Design review of the part built by this model. Coordinates are the model's own, in mm. Give positions to 0.01 mm unless a question says otherwise; leave off trailing zeros. Write each loop counter-clockwise with the first axis right and the second up, starting at its lowest first coordinate (ties: lowest second). Pieces come first, ordered by that corner, then holes. Notation, with made-up numbers: (-40, 30) -> (-15, 30) arc R14 ccw to (-15, 37) -> close; hole circle Ø11 at (15, 74). An arc over 180 degrees is marked (long way). Answer as a JSON object with one key per item and string values.
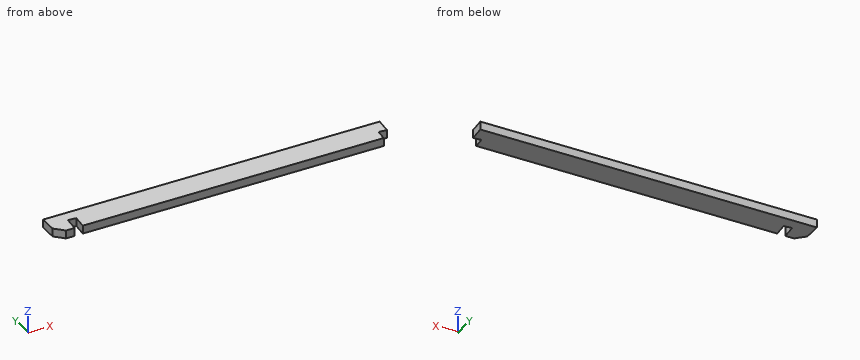
```python
from build123d import *

# Parameters (mm, degrees)
SKETCH1_W           = 47
SKETCH1_H           = 150
BOSS_EXTRUDE1_DEPTH = 1955
CUT_EXTRUDE1_DEPTH  = 1958.002554929
CHAMFER1_SIZE       = 50
CUT_EXTRUDE2_DEPTH  = 1958.002554929
CUT_EXTRUDE3_DEPTH  = 1958.002554929


with BuildPart() as part:
    # Sketch1 → Boss-Extrude1 (new body)
    with BuildSketch(Plane(origin=(0, 0, 0), x_dir=(0, 0, -1), z_dir=(1, 0, 0))):
        Rectangle(SKETCH1_W, SKETCH1_H)
    extrude(amount=BOSS_EXTRUDE1_DEPTH)

    # Sketch2 → Cut-Extrude1 (cut, through all)
    with BuildSketch(Plane.XY.offset(23.5)):
        Polygon((100, -75), (107.357474636, 9.096319909), (154.178625447, 5), (147.179532365, -75), align=None)
    extrude(amount=-CUT_EXTRUDE1_DEPTH, mode=Mode.SUBTRACT)

    # Chamfer1
    chamfer1_edges = [part.edges().sort_by_distance(p)[0] for p in [
        (0, -75, 0),
    ]]
    chamfer(chamfer1_edges, length=CHAMFER1_SIZE)

    # Sketch3 → Cut-Extrude2 (cut, through all)
    with BuildSketch(Plane(origin=(0, 0, -23.5), x_dir=(-1, 0, 0), z_dir=(0, 0, -1))):
        Polygon((-1955, 75), (-1941.876700471, -75), (-1955, -75), align=None)
    extrude(amount=-CUT_EXTRUDE2_DEPTH, mode=Mode.SUBTRACT)

    # Sketch4 → Cut-Extrude3 (cut, through all)
    with BuildSketch(Plane.XY.offset(23.5)):
        Polygon((1947.126020283, -15), (1900.304869472, -10.903680091), (1894.697168107, -75), (1941.876700471, -75), align=None)
    extrude(amount=-CUT_EXTRUDE3_DEPTH, mode=Mode.SUBTRACT)


solid = part.part
```
(1) For line 1 along X through (y, z) = (-39, 11); line 2 along X through (y, z) = (-34.5, 7.5); line 3 along X through (y, z) = (33, 19), list the stretches that pass through material, from the lowest coordinate up.
Here are the results:
{"line 1": "x = 14 to 103.15, 150.33 to 1897.85", "line 2": "x = 9.5 to 103.54, 150.72 to 1898.24", "line 3": "x = 0 to 1951.33"}
(2) We need section A-A, the plane z = 2.5. State the section outline as (x, y) points.
Here are the results:
{"outline": "(0, -25) -> (50, -75) -> (100, -75) -> (107.36, 9.1) -> (154.18, 5) -> (147.18, -75) -> (1894.7, -75) -> (1900.3, -10.9) -> (1947.13, -15) -> (1955, 75) -> (0, 75) -> close"}
(3) Clearance check with a flat-ended pin moving along its axis: pin 1 (1.5 mm diameter, centred on y = -53, z = -18.5, fed in from -X). State where the tip first meets the part, or that it passes through.
Here are the results:
{"pin 1": "stops at x = 27.25"}
